from build123d import *

# Parameters (mm, degrees)
CROQUIS1_R              = 1.25
SALIENTE_EXTRUIR1_DEPTH = 6
CROQUIS2_R              = 2.25
SALIENTE_EXTRUIR2_DEPTH = 2.5
CORTAR_EXTRUIR1_DEPTH   = 1.5
REDONDEO1_R             = 0.35


with BuildPart() as part:
    # Croquis1 → Saliente-Extruir1 (new body)
    with BuildSketch(Plane.XY):
        Circle(CROQUIS1_R)
    extrude(amount=SALIENTE_EXTRUIR1_DEPTH)

    # Croquis2 → Saliente-Extruir2 (add)
    with BuildSketch(Plane(origin=(0, 0, 0), x_dir=(-1, 0, 0), z_dir=(0, 0, -1))):
        Circle(CROQUIS2_R)
    extrude(amount=SALIENTE_EXTRUIR2_DEPTH)

    # Croquis3 → Cortar-Extruir1 (cut)
    with BuildSketch(Plane(origin=(0, 0, -2.5), x_dir=(-1, 0, 0), z_dir=(0, 0, -1))):
        Polygon((0, -1.154700538), (1, -0.577350269), (1, 0.577350269), (0, 1.154700538), (-1, 0.577350269), (-1, -0.577350269), align=None)
    extrude(amount=-CORTAR_EXTRUIR1_DEPTH, mode=Mode.SUBTRACT)

    # Redondeo1
    redondeo1_edges = [part.edges().sort_by_distance(p)[0] for p in [
        (2.25, 0, -2.5),
    ]]
    fillet(redondeo1_edges, radius=REDONDEO1_R)


solid = part.part
Verification items for the finished model (mm, model axes). A direction names the side the tool comes from. Coordinates: 2 decimals unless noted, no trailing zeros. Order: outer loops, then holes, each group sorted by start corner. A loop starts at its lowest first (then second) coordinate and runs counter-clockwise, first axis right, second up. Notation, with made-up numbers: M 37,82.25 L 71,82.25 A22 ccw 71,113.25 Z; hole C 75.5,11 d5. An arc over 180 degrees is marked long. Return JSON: item names as keys, results as strings.
1) Gauge pin test, flat ends, axial feed: pin 1 (2 mm diameter, centred on x = 0, y = -0.5, fed in from -Z); pin 2 (1 mm diameter, centred on x = 1, z = -1, fed in from -Y). Record the tip position at first contact, or that the pin passes through.
Answer list:
{"pin 1": "z = -2.5", "pin 2": "y = -2.19"}
2) Access from +Z, -Z, +X, -X, +Y, -Y to the whole of each face (thin tool, end or side, straight path). Record for faces 1 (the flat face through (0.49, 0.87, -1.76)), 2 (the flat face through (0, 0, 6)), 3 (the cylindrical face through (-0.27, -1.22, 2.96)).
Answer list:
{"face 1": "-Z", "face 2": "+Z, +X, -X, +Y, -Y", "face 3": "+Z"}
3) Cross-section at A-A, the plane y = 0. Record the boundary of the cut face in (x, z).
Answer list:
{"outline": "M -2.25,-2.15 A0.35 ccw -1.9,-2.5 L -1,-2.5 L -1,-1 L 1,-1 L 1,-2.5 L 1.9,-2.5 A0.35 ccw 2.25,-2.15 L 2.25,0 L 1.25,0 L 1.25,6 L -1.25,6 L -1.25,0 L -2.25,0 Z"}
4) Cross-section at B-B, the plane z = 4.5. Record the boundary of the cut face in (x, y), and give its area (3 significant figures).
Answer list:
{"outline": "C 0,0 d2.5", "area": "4.91 mm2"}
5) Release check for a two-part mould opening along Y. For faces 4 (the flat face through (-1, -1, -2.5)), 5 (the flat face through (0.51, -0.86, -1.76)), 6 (the flat face through (1, 0, -2)), 7 (the cylindrical face through (0.29, 2.23, -1.06)) record: +Y half, -Y half, draft (parallel to the pull), parting line (faces both ways), or undercut.
Answer list:
{"face 4": "draft", "face 5": "undercut", "face 6": "undercut", "face 7": "parting line"}
6) Thickness scan on L1, parallel to Z at x = -1.35, y = 0.7; L2, parallel to Z at x = -0.1, y = -0.5; L3, parallel to Y at x = 1.2, z = -1.5. Record the ranges inside material, lowest first. Write a range as [from, to].
Answer list:
{"L1": "[-2.5, 0]", "L2": "[-1, 6]", "L3": "[-1.9, 1.9]"}
